```python
from build123d import *

# Parameters (mm, degrees)
SKETCH1_W           = 170
SKETCH1_H           = 160
SKETCH1_R           = 29
BOSS_EXTRUDE1_DEPTH = 6.35
SKETCH2_W           = 50.8
SKETCH2_H           = 50.8
CUT_EXTRUDE1_DEPTH  = 234.538695937
FILLET1_R           = 10
CUT_EXTRUDE2_DEPTH  = 234.538695937


with BuildPart() as part:
    # Sketch1 → Boss-Extrude1 (new body)
    with BuildSketch(Plane(origin=(0, 0, 0), x_dir=(1, 0, 0), z_dir=(0, 1, 0))):
        with Locations((85, 80)):
            Rectangle(SKETCH1_W, SKETCH1_H)
        with Locations(Location((110, 100, 0), (0, 0, 270))):
            Circle(SKETCH1_R, mode=Mode.SUBTRACT)
    extrude(amount=BOSS_EXTRUDE1_DEPTH)

    # Sketch2 → Cut-Extrude1 (cut, through all)
    with BuildSketch(Plane(origin=(0, 6.35, 0), x_dir=(1, 0, 0), z_dir=(0, 1, 0))):
        with Locations((25.4, 25.4)):
            Rectangle(SKETCH2_W, SKETCH2_H)
    extrude(amount=-CUT_EXTRUDE1_DEPTH, mode=Mode.SUBTRACT)

    # Fillet1
    fillet1_edges = [part.edges().sort_by_distance(p)[0] for p in [
        (0, 3.175, -50.8),
        (50.8, 3.175, -50.8),
        (50.8, 3.175, 0),
        (0, 3.175, -160),
        (170, 3.175, -160),
        (170, 3.175, 0),
    ]]
    fillet(fillet1_edges, radius=FILLET1_R)

    # Sketch3 → Cut-Extrude2 (cut, through all)
    with BuildSketch(Plane(origin=(0, 6.35, 0), x_dir=(1, 0, 0), z_dir=(0, 1, 0))):
        with BuildLine():
            Line((63.698729811, 80.196152423), (72.358983849, 85.196152423))
            ThreePointArc((72.358983849, 85.196152423), (80.555136271, 83), (78.358983849, 74.803847577))
            Line((78.358983849, 74.803847577), (69.698729811, 69.803847577))
            ThreePointArc((69.698729811, 69.803847577), (61.502577388, 72), (63.698729811, 80.196152423))
        make_face()
        with BuildLine():
            Line((150.301270189, 69.803847577), (141.641016151, 74.803847577))
            ThreePointArc((141.641016151, 74.803847577), (139.444863729, 83), (147.641016151, 85.196152423))
            Line((147.641016151, 85.196152423), (156.301270189, 80.196152423))
            ThreePointArc((156.301270189, 80.196152423), (158.497422612, 72), (150.301270189, 69.803847577))
        make_face()
        with BuildLine():
            Line((116, 150), (116, 140))
            ThreePointArc((116, 140), (110, 134), (104, 140))
            Line((104, 140), (104, 150))
            ThreePointArc((104, 150), (110, 156), (116, 150))
        make_face()
    extrude(amount=-CUT_EXTRUDE2_DEPTH, mode=Mode.SUBTRACT)


solid = part.part
```
Geometry check sheet. Reference: the model listing, model coordinates, mm. A direction names the side the tool comes from. Coordinates: 2 decimals unless noted, no trailing zeros. Write each loop counter-clockwise with the first axis right and the second up, starting at its lowest first coordinate (ties: lowest second). Pieces come first, ordered by that corner, then holes. Notation, with made-up numbers: M 74.5,-12 L 126.5,-12 A36 cw 126.5,22 Z; hole C 23.25,-38 d7. An arc over 180 degrees is marked long. One line per item, written item: value. Start each with the question number.
(1) Sectioned sample at A-A, the plane x = 110. Enter the section's corners in (y, z).
(2) Scan lines: line 1 along X through (y, z) = (5, -100); line 2 along X through (y, z) = (5, -81); line 3 along X through (y, z) = (1.75, -21). Record each from-to range of solid material in increasing order. Write a range as [from, to].
(3) Sectioned sample at C-C, the plane y = 5. Enter the section's corners in (x, z), and give its area (3 significant figures).
(4) Release check for a two-part mould opening along Z. For faces 4 (the face through (2.85, 3.13, -53.81)), 5 (the face through (61.57, 3.219, -71.886)), 6 (the face through (110, 3, -134)), 7 (the face through (170, 3, -79)) record: released by +Z, released by -Z, zero draft, split by the parting line, or undercut.
(5) Depth check by flat-ended pin: pin 1 (1.9 mm diameter, centred on y = 2.5, z = -23, fed in from -X); pin 2 (2 mm diameter, centred on x = 92, z = -136.5, fed in from -Y). Enter the tip coordinate at first touch or a pass-through.
(6) Tool access check on faces 1 (the face through (25, 3, -50.8)), 2 (the face through (2.85, 3.22, -156.99)), 3 (the face through (104, 3, -145)). Record the directions out of +Z, -Z, +X, -X, +Y, -Y that give a thin tool (end or side, any length) a straight path to the whole face; none if there is none.
(7) Sectioned sample at D-D, the plane x = 24. Enter the section's corners in (y, z), and give its area (3 significant figures).
(8) Sectioned sample at B-B, the plane z = -100. Enter the section's corners in (x, y).
Filled sheet:
1. outline: M 0,-160 L 6.35,-160 L 6.35,-156 L 0,-156 Z; M 0,-134 L 6.35,-134 L 6.35,-129 L 0,-129 Z; M 0,-71 L 6.35,-71 L 6.35,0 L 0,0 Z
2. line 1: [0, 81], [139, 170]
2. line 2: [0, 65.09], [81.28, 88.09], [131.91, 138.72], [154.91, 170]
2. line 3: [50.8, 170]
3. outline: M 0,-150 A10 ccw 10,-160 L 160,-160 A10 ccw 170,-150 L 170,-10 A10 ccw 160,0 L 60.8,0 A10 ccw 50.8,-10 L 50.8,-40.8 A10 cw 40.8,-50.8 L 10,-50.8 A10 ccw 0,-60.8 Z; hole M 63.7,-80.2 L 72.36,-85.2 A6 ccw 78.36,-74.8 L 69.7,-69.8 A6 ccw Z; hole C 110,-100 d58; hole M 104,-150 A6 ccw 116,-150 L 116,-140 A6 ccw 104,-140 Z; hole M 141.64,-74.8 A6 ccw 147.64,-85.2 L 156.3,-80.2 A6 ccw 150.3,-69.8 Z
3. area: 21,200 mm²
4. face 4: released by +Z
4. face 5: undercut
4. face 6: undercut
4. face 7: zero draft
5. pin 1: x = 50.8
5. pin 2: y = 0
6. face 1: +Z, -X, +Y, -Y
6. face 2: -Z, -X, +Y, -Y
6. face 3: +Y, -Y
7. outline: M 0,-160 L 6.35,-160 L 6.35,-50.8 L 0,-50.8 Z
7. area: 693 mm²
8. outline: M 0,0 L 81,0 L 81,6.35 L 0,6.35 Z; M 139,0 L 170,0 L 170,6.35 L 139,6.35 Z
